```python
from build123d import *

# Parameters (mm, degrees)
SKETCH1_W           = 41.2
SKETCH1_H           = 21
SKETCH1_R           = 4.05
SKETCH1_R_2         = 1.5
BOSS_EXTRUDE1_DEPTH = 2
SKETCH2_W           = 2
SKETCH2_H           = 21
BOSS_EXTRUDE2_DEPTH = 28.2
SKETCH3_R           = 1.5
SKETCH3_R_2         = 4.25
CUT_EXTRUDE1_DEPTH  = 53.151030671
CUT_EXTRUDE2_DEPTH  = 53.151030671
FILLET1_R           = 2


with BuildPart() as part:
    # Sketch1 → Boss-Extrude1 (new body)
    with BuildSketch(Plane(origin=(0, 0, 0), x_dir=(1, 0, 0), z_dir=(0, 1, 0))):
        Rectangle(SKETCH1_W, SKETCH1_H)
        with Locations(Location((0, 0, 0), (0, 0, 270))):
            Circle(SKETCH1_R, mode=Mode.SUBTRACT)
        with Locations(Location((0, 7, 0), (0, 0, 270))):
            Circle(SKETCH1_R_2, mode=Mode.SUBTRACT)
        with Locations(Location((7, 0, 0), (0, 0, 270))):
            Circle(SKETCH1_R_2, mode=Mode.SUBTRACT)
        with Locations(Location((0, -7, 0), (0, 0, 270))):
            Circle(SKETCH1_R_2, mode=Mode.SUBTRACT)
        with Locations(Location((-7, 0, 0), (0, 0, 270))):
            Circle(SKETCH1_R_2, mode=Mode.SUBTRACT)
        with Locations(Location((6, -8, 0), (0, 0, 270))):
            Circle(SKETCH1_R_2, mode=Mode.SUBTRACT)
        with Locations(Location((6, 8, 0), (0, 0, 270))):
            Circle(SKETCH1_R_2, mode=Mode.SUBTRACT)
        with Locations(Location((-6, 8, 0), (0, 0, 270))):
            Circle(SKETCH1_R_2, mode=Mode.SUBTRACT)
        with Locations(Location((-6, -8, 0), (0, 0, 270))):
            Circle(SKETCH1_R_2, mode=Mode.SUBTRACT)
    extrude(amount=BOSS_EXTRUDE1_DEPTH)

    # Sketch2 → Boss-Extrude2 (add)
    with BuildSketch(Plane(origin=(0, 2, 0), x_dir=(1, 0, 0), z_dir=(0, 1, 0))):
        with Locations((-19.6, 0)):
            Rectangle(SKETCH2_W, SKETCH2_H)
        with Locations((19.6, 0)):
            Rectangle(SKETCH2_W, SKETCH2_H)
    extrude(amount=BOSS_EXTRUDE2_DEPTH)

    # Sketch3 → Cut-Extrude1 (cut, through all)
    with BuildSketch(Plane.ZY.offset(20.6)):
        with Locations((-7, 25.9)):
            Circle(SKETCH3_R)
        with Locations((0, 18.9)):
            Circle(SKETCH3_R)
        with Locations((7, 25.9)):
            Circle(SKETCH3_R)
        with Locations((0, 25.9)):
            Circle(SKETCH3_R_2)
    extrude(amount=-CUT_EXTRUDE1_DEPTH, mode=Mode.SUBTRACT)

    # Sketch4 → Cut-Extrude2 (cut, through all)
    with BuildSketch(Plane.ZY.offset(20.6)):
        with BuildLine():
            Line((-10.5, 25.944077053), (-10.5, 30.2))
            Line((-10.5, 30.2), (10.5, 30.2))
            Line((10.5, 30.2), (10.5, 25.944076968))
            ThreePointArc((10.5, 25.944076968), (7.374885716, 29.069191252), (4.249771432, 25.944076968))
            ThreePointArc((4.249771432, 25.944076968), (0, 21.69430542), (-4.249771432, 25.944076968))
            ThreePointArc((-4.249771432, 25.944076968), (-7.374885673, 29.069191338), (-10.5, 25.944077053))
        make_face()
    extrude(amount=-CUT_EXTRUDE2_DEPTH, mode=Mode.SUBTRACT)

    # Fillet1
    fillet1_edges = [part.edges().sort_by_distance(p)[0] for p in [
        (20.6, 0, 0),
        (-20.6, 0, 0),
    ]]
    fillet(fillet1_edges, radius=FILLET1_R)


solid = part.part
```
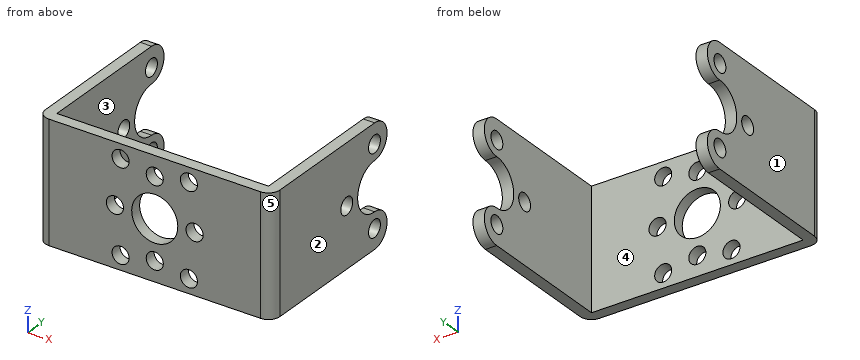
Geometry: final body of the model. Coordinates: model frame, mm. Face numbers are marked on the shaded views. A direction names the side the tool comes from. Round coordinates to 2 decimals unless told otherwise and drop trailing zeros. Write each loop counter-clockwise with the first axis right and the second up, starting at its lowest first coordinate (ties: lowest second). Pieces come first, ordered by that corner, then holes. Notation, with made-up numbers: M -34,59.5 L 23,59.5 A11 cw 23,76.5 Z; hole C 63.5,-23 d10. An arc over 180 degrees is marked long. Answer in a Markdown table with one row per item. Add a question column.
(1) Reachability of the marked faces 4 and 5 from +Z, -Z, +X, -X, +Y, -Y: full face, straight path, thin tool, end or side. Return the list, or none.
(2) Cut plane B-B, the plane y = 18.9. Return the cut outline in (x, z), then the cut area to 3 significant figures.
(3) Cut plane A-A, the plane x = 0. Return the cut outline in (y, z).
(4) Draft query along X for the marked faces 1, 2 and 3. Return one class per face: pulls with the +X half, pulls with the -X half, needs draft (parallel to the pull), parting line crosses it, or undercut.
(5) Cut plane C-C, the plane z = 8. Give the number of separate pieces and of enclosed holes in the cut face, then the cut area to 3 significant figures.
(6) Contact query for a flat-ended pin moving along its axis: pin 1 (6.5 mm diameter, centred on x = 0, z = 3, fed in from +Y). Output: stop coordinate, or through.
(7) Ray query, L1, parallel to X at y = 1.2, z = 0; L2, parallel to X at y = 0.55, z = -8; L3, parallel to X at y = 7.25, z = -7.75. Return the intervals inside material, ascending.
(8) Cut plane D-D, the plane z = -2. Return the cut outline in (x, y).
Established:
| question | item | result |
|---|---|---|
| 1 | face 4 | +Z, -Z, +Y |
| 1 | face 5 | +Z, -Z, +X, -Y |
| 2 | outline | M -20.6,-10.5 L -18.6,-10.5 L -18.6,-1.5 L -20.6,-1.5 Z; M -20.6,1.5 L -18.6,1.5 L -18.6,10.5 L -20.6,10.5 Z; M 18.6,-10.5 L 20.6,-10.5 L 20.6,-1.5 L 18.6,-1.5 Z; M 18.6,1.5 L 20.6,1.5 L 20.6,10.5 L 18.6,10.5 Z |
| 2 | area | 72.0 mm² |
| 3 | outline | M 0,-10.5 L 2,-10.5 L 2,-8.5 L 0,-8.5 Z; M 0,-5.5 L 2,-5.5 L 2,-4.05 L 0,-4.05 Z; M 0,4.05 L 2,4.05 L 2,5.5 L 0,5.5 Z; M 0,8.5 L 2,8.5 L 2,10.5 L 0,10.5 Z |
| 4 | face 1 | pulls with the -X half |
| 4 | face 2 | pulls with the +X half |
| 4 | face 3 | undercut |
| 5 | separate pieces | 6 |
| 5 | enclosed holes | 0 |
| 5 | area | 163 mm² |
| 6 | pin 1 | y = 2 |
| 7 | L1 | -20.43 to -8.5, -5.5 to -4.05, 4.05 to 5.5, 8.5 to 20.43 |
| 7 | L2 | -19.98 to -7.5, -4.5 to -1.12, 1.12 to 4.5, 7.5 to 19.98 |
| 7 | L3 | -20.6 to -18.6, 18.6 to 20.6 |
| 8 | outline | M -20.6,2 A2 ccw -18.6,0 L -3.52,0 L -3.52,2 L -18.6,2 L -18.6,22.15 L -20.6,22.15 Z; M 3.52,0 L 18.6,0 A2 ccw 20.6,2 L 20.6,22.15 L 18.6,22.15 L 18.6,2 L 3.52,2 Z |
